```python
from build123d import *

# Parameters (mm, degrees)
F0_W     = 50.8
F0_H     = 24.7
F1_DEPTH = 1
F2_R     = 1.503447
F3_DEPTH = 25
F5_DEPTH = 25


with BuildPart() as f1:
    # F0 (on Top) → F1 (new body)
    with BuildSketch(Plane.XY):
        Rectangle(F0_W, F0_H)
    extrude(amount=F1_DEPTH)

    # F2 (on face) → F3 (cut)
    with BuildSketch(Plane.XY.offset(1)):
        with Locations((20.966841, 0)):
            Circle(F2_R)
    extrude(amount=-F3_DEPTH, mode=Mode.SUBTRACT)

    # F4 (on face) → F5 (cut)
    with BuildSketch(Plane(origin=(0, 0, 0), x_dir=(1, 0, 0), z_dir=(0, 0, -1))):
        Polygon((-13.518144, 21.329358), (-20.957662, 12.35), (-13.518144, 2.8125), (-4.808467, 12.35), align=None)
    extrude(amount=-F5_DEPTH, mode=Mode.SUBTRACT)


solid = f1.part
```
Verification items for the finished model (mm, model axes). Give positions to 0.01 mm unless a question says otherwise; leave off trailing zeros. Loops run counter-clockwise (first coordinate to the right, second up) from the corner with the lowest first, then second, coordinate; pieces in that order, holes last.
1. Section check B-B, the plane z = 0.7. Enter the section's corners in (x, y), then the cut area to 3 significant figures.
2. Section check D-D, the plane x = -20. Enter the section's corners in (y, z).
3. Section check C-C, the plane x = 22. Enter the section's corners in (y, z), then the cut area to 3 significant figures.
4. Mould release check, pull along X, two halves, no side actions. Record for faces 1 (the flat face through (0, 0, 1)), 2 (the flat face through (-25.4, -0.2, 0.5)), 3 (the flat face through (-9.224, -7.514, 0.493)), 4 (the flat face through (-17.29, -7.65, 0.49)): released by +X, released by -X, zero draft, split by the parting line, or undercut.
5. Thickness scan on line 1 (X direction, y = -11, z = 0.9); line 2 (X direction, y = -8.75, z = 0.3); line 3 (Y direction, x = -8, z = 0.65). Record the ranges inside material, lowest first.
6. Section check A-A, the plane y = 0. Enter the section's corners in (x, z), then the cut area to 3 significant figures.
Geometry says:
1. outline: (-25.4, -12.35) - (-20.96, -12.35) - (-13.52, -2.81) - (-4.81, -12.35) - (25.4, -12.35) - (25.4, 12.35) - (-25.4, 12.35) - close; hole circle Ø3.01 at (20.97, 0)
1. area: 1,170 mm2
2. outline: (-11.12, 0) - (12.35, 0) - (12.35, 1) - (-11.12, 1) - close
3. outline: (-12.35, 0) - (-1.09, 0) - (-1.09, 1) - (-12.35, 1) - close; (1.09, 0) - (12.35, 0) - (12.35, 1) - (1.09, 1) - close
3. area: 22.5 mm2
4. face 1: zero draft
4. face 2: released by -X
4. face 3: undercut
4. face 4: undercut
5. line 1: x = -25.4 to -19.9, -6.04 to 25.4
5. line 2: x = -25.4 to -18.15, -8.1 to 25.4
5. line 3: y = -8.86 to 12.35
6. outline: (-25.4, 0) - (19.46, 0) - (19.46, 1) - (-25.4, 1) - close; (22.47, 0) - (25.4, 0) - (25.4, 1) - (22.47, 1) - close
6. area: 47.8 mm2
